The model under review builds one solid part; all positions refer to its coordinate system, in mm. Give positions to 0.01 mm unless a question says otherwise; leave off trailing zeros. Order: outer loops, then holes, each group sorted by start corner. A loop starts at its lowest first (then second) coordinate and runs counter-clockwise, first axis right, second up.
```python
from build123d import *

# Parameters (mm, degrees)
F0_W     = 127
F0_H     = 127
F0_R     = 1.778
F1_DEPTH = 2.921


with BuildPart() as f1:
    # F0 (on Top) → F1 (new body)
    with BuildSketch(Plane.XY):
        with Locations((63.5, 63.5)):
            Rectangle(F0_W, F0_H)
        with Locations((6.35, 6.35)):
            Circle(F0_R, mode=Mode.SUBTRACT)
        with Locations((18.598719, 18.598719)):
            Circle(F0_R, mode=Mode.SUBTRACT)
        with Locations((49.8475, 49.8475)):
            Circle(F0_R, mode=Mode.SUBTRACT)
        with Locations((120.65, 6.35)):
            Circle(F0_R, mode=Mode.SUBTRACT)
        with Locations((108.401281, 18.598719)):
            Circle(F0_R, mode=Mode.SUBTRACT)
        with BuildLine():
            Line((53.192581, 72.294635), (53.192581, 82.55))
            Line((53.192581, 82.55), (73.512581, 82.55))
            Line((73.512581, 82.55), (73.512581, 72.607131))
            ThreePointArc((73.512581, 72.607131), (76.442887, 68.12262), (77.47, 62.865))
            ThreePointArc((77.47, 62.865), (76.442887, 57.60738), (73.512581, 53.122869))
            Line((73.512581, 53.122869), (73.512581, 15.335365))
            Line((73.512581, 15.335365), (53.192581, 15.335365))
            Line((53.192581, 15.335365), (53.192581, 53.435365))
            ThreePointArc((53.192581, 53.435365), (49.53, 62.865), (53.192581, 72.294635))
        make_face(mode=Mode.SUBTRACT)
        with Locations((77.1525, 49.8475)):
            Circle(F0_R, mode=Mode.SUBTRACT)
        with Locations((49.8475, 75.8825)):
            Circle(F0_R, mode=Mode.SUBTRACT)
        with Locations((18.598719, 108.401281)):
            Circle(F0_R, mode=Mode.SUBTRACT)
        with Locations((6.35, 120.65)):
            Circle(F0_R, mode=Mode.SUBTRACT)
        with Locations((77.1525, 75.8825)):
            Circle(F0_R, mode=Mode.SUBTRACT)
        with Locations((108.401281, 108.401281)):
            Circle(F0_R, mode=Mode.SUBTRACT)
        with Locations((120.65, 120.65)):
            Circle(F0_R, mode=Mode.SUBTRACT)
    extrude(amount=F1_DEPTH)


solid = f1.part
```
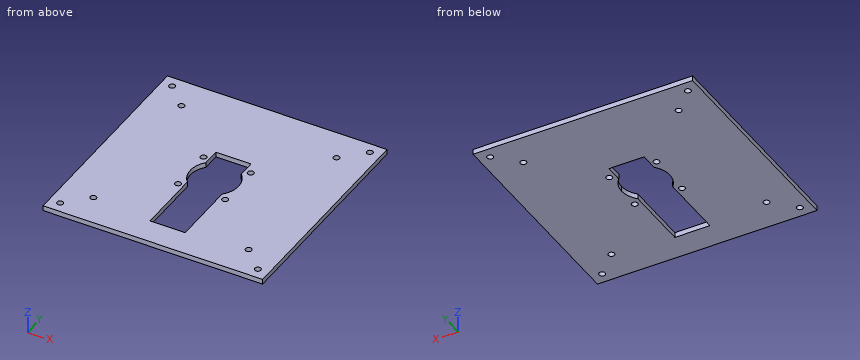
1. Insertion check: pin 1 (4 mm diameter, centred on x = 104.5, y = 44, fed in from -Z); pin 2 (3 mm diameter, centred on x = 120.65, y = 120.65, fed in from -Z). Each pin has a flat end and moves straight along its axis. Give the tip position at first contact, or say it passes through.
2. To check wall thickness, follow line 1 (Y direction, x = 120.65, z = 0.8); line 2 (X direction, y = 28.5, z = 1.45); line 3 (Y direction, x = 20, z = 1.55). State the ranges of each line that lie inside material, in increasing order.
3. Take a section at D-D (z = 0.95). Count the separate pieces of the cut face and the enclosed holes in it, and give its area (3 significant figures).
4. Take a section at A-A (y = 120.65). Write out the cut boundary in (x, z), and give its area (3 significant figures).
5. Take a section at C-C (y = 41). Write out the cut boundary in (x, z).
Answer:
1. pin 1: stops at z = 0
1. pin 2: passes through
2. line 1: y = 0 to 4.57, 8.13 to 118.87, 122.43 to 127
2. line 2: x = 0 to 53.19, 73.51 to 127
2. line 3: y = 0 to 17.5, 19.69 to 107.31, 109.5 to 127
3. separate pieces: 1
3. enclosed holes: 13
3. area: 14,500 mm2
4. outline: (0, 0) - (4.57, 0) - (4.57, 2.92) - (0, 2.92) - close; (8.13, 0) - (118.87, 0) - (118.87, 2.92) - (8.13, 2.92) - close; (122.43, 0) - (127, 0) - (127, 2.92) - (122.43, 2.92) - close
4. area: 350 mm2
5. outline: (0, 0) - (53.19, 0) - (53.19, 2.92) - (0, 2.92) - close; (73.51, 0) - (127, 0) - (127, 2.92) - (73.51, 2.92) - close
